```python
from build123d import *

# Parameters (mm, degrees)
CROQUIS1_W              = 78
CROQUIS1_H              = 20.5
SALIENTE_EXTRUIR1_DEPTH = 21.5
VACIADO1_T              = -2
CROQUIS2_W              = 74
CROQUIS2_H              = 12.5
CORTAR_EXTRUIR1_DEPTH   = 41.5


with BuildPart() as part:
    # Croquis1 → Saliente-Extruir1 (new body)
    with BuildSketch(Plane(origin=(0, 0, 0), x_dir=(1, 0, 0), z_dir=(0, 1, 0))):
        Rectangle(CROQUIS1_W, CROQUIS1_H)
    extrude(amount=SALIENTE_EXTRUIR1_DEPTH)

    # Vaciado1
    vaciado1_openings = [part.faces().sort_by_distance(p)[0] for p in [
        (0, 21.5, 0),
    ]]
    offset(amount=VACIADO1_T, openings=vaciado1_openings, kind=Kind.INTERSECTION)

    # Croquis2 → Cortar-Extruir1 (cut)
    with BuildSketch(Plane.XY.offset(10.25)):
        with Locations((0, 15.25)):
            Rectangle(CROQUIS2_W, CROQUIS2_H)
    extrude(amount=-CORTAR_EXTRUIR1_DEPTH, mode=Mode.SUBTRACT)


solid = part.part
```
Read the model definition and answer for the solid it produces. Units are mm, in the model's axes. A direction names the side the tool comes from. Coordinates: 2 decimals unless noted, no trailing zeros. Write each loop counter-clockwise with the first axis right and the second up, starting at its lowest first coordinate (ties: lowest second). Pieces come first, ordered by that corner, then holes. Notation, with made-up numbers: (83, -21.75) - (109, -21.75) arc R16 ccw to (109, 1.25) - close; hole circle Ø11 at (61.25, 51). An arc over 180 degrees is marked (long way). Answer as a JSON object with one key per item and string values. Group by question number.
1. Each of these flat-tipped pins is pushed along its axis until it touches: P1, Ø6, axis at x = 29.5, y = 14.5, coming from the -Z side; P2, Ø6, axis at x = 5, z = 8, coming from the -Y side; P3, Ø4, axis at x = 27, z = -0.5, coming from the +Y side; P4, Ø1, axis at x = 7, z = 9.5, coming from the +Y side. Where does it stop, or does it pass through?
2. A cutting plane is placed at B-B (x = 33). Determine the outline of the cut face in (y, z), plus the area to 3 significant figures.
3. The mould has two halves that part along Z. Classify faces 4 (the flat face through (-1, 3, 10.25)), 5 (the flat face through (-1, 5, 8.25)), 6 (the flat face through (39, 11, 0)): +Z half, -Z half, draft (parallel to the pull), parting line (faces both ways), or undercut.
4. Which of the six approach directions +Z, -Z, +X, -X, +Y, -Y give full straight-line access (tool end or side, diameter ignored) to faces 1 (the flat face through (-1, 9, 9)), 2 (the flat face through (38, 21.5, 0)), 3 (the flat face through (-1, 2, 0))?
5. A cutting plane is placed at A-A (y = 11.25). Determine the outline of the cut face in (x, z).
6. A cutting plane is placed at C-C (z = -6.75). Determine the outline of the cut face in (x, y).
7. Consider L1, parallel to X at y = 6.25, z = -2.25; L2, parallel to Z at x = -9, y = 5.75; L3, parallel to Y at x = 35.5, z = 0.5. Determine where each line is inside the solid, lowest interval first. Write a range as [from, to].
Worked out:
{
 "1": {"P1": "passes through", "P2": "stops at y = 0", "P3": "stops at y = 2", "P4": "stops at y = 9"},
 "2": {"outline": "(0, -10.25) - (9, -10.25) - (9, -8.25) - (2, -8.25) - (2, 8.25) - (9, 8.25) - (9, 10.25) - (0, 10.25) - close", "area": "69.0 mm²"},
 "3": {"face 4": "+Z half", "face 5": "undercut", "face 6": "draft"},
 "4": {"face 1": "+Z, -Z, +Y", "face 2": "+Z, -Z, +X, -X, +Y", "face 3": "+Y"},
 "5": {"outline": "(-39, -10.25) - (-37, -10.25) - (-37, 10.25) - (-39, 10.25) - close; (37, -10.25) - (39, -10.25) - (39, 10.25) - (37, 10.25) - close"},
 "6": {"outline": "(-39, 0) - (39, 0) - (39, 21.5) - (37, 21.5) - (37, 2) - (-37, 2) - (-37, 21.5) - (-39, 21.5) - close"},
 "7": {"L1": "x = [-39, -37], [37, 39]", "L2": "z = [-10.25, -8.25], [8.25, 10.25]", "L3": "y = [0, 2]"}
}
